Part model, mm, in its own coordinate system. A direction names the side the tool comes from. Give positions to 0.01 mm unless a question says otherwise; leave off trailing zeros. Order: outer loops, then holes, each group sorted by start corner. A loop starts at its lowest first (then second) coordinate and runs counter-clockwise, first axis right, second up. Notation, with made-up numbers: (39.25, 21) - (62.25, 21) arc R11 cw to (62.25, 27) - close; hole circle Ø9 at (85, -12.75). An arc over 180 degrees is marked (long way). One line per item, written item: value.
Autodesk Inventor part; units mm, degrees
ref_plane "YZ Plane" through (0, 0, 0) normal (1, 0, 0) x (0, 1, 0)
ref_plane "XZ Plane" through (0, 0, 0) normal (0, 1, 0) x (-1, 0, 0)
ref_plane "XY Plane" through (0, 0, 0) normal (0, 0, 1) x (1, 0, 0)
sketch "Sketch1" plane through (0, 0, 0) normal (0, 1, 0) x (-1, 0, 0)
  line L0 (18.2162, 77.2548) -> (-57.9838, 77.2548)
  line L1 (-57.9838, 77.2548) -> (-57.9838, -24.3452)
  line L2 (-57.9838, -24.3452) -> (18.2162, -24.3452)
  line L3 (18.2162, -24.3452) -> (18.2162, 77.2548)
  point P0 (0, 0)
  dimension "d0" = 101.6
  dimension "d1" = 76.2
extrude "Extrusion1" add sketch "Sketch1" along normal blind 12.7
sketch "Sketch2" plane through (57.9838, 0, -24.3452) normal (0, 0, -1) x (-1, 0, 0)
  line L0 (0, 0) -> (0, -203.2)
  line L1 (0, -203.2) -> (76.2, -203.2)
  line L2 (0, 0) -> (76.2, 0)
  line L3 (76.2, -203.2) -> (76.2, 0)
  line L4 (0, 12.7) -> (76.2, 12.7)
  line L5 (0, 0) -> (0, 12.7)
  line L6 (0, 12.7) -> (76.2, 12.7)
  line L7 (76.2, 12.7) -> (76.2, 0)
  point P0 (57.9838, 0)
  dimension "d4" = 90
  dimension "d5" = 203.2
extrude "Extrusion2" add sketch "Sketch2" along normal blind 12.7
sketch "Sketch3" plane through (-18.2162, 0, 77.2548) normal (0, 0, 1) x (1, 0, 0)
  line L0 (0, 0) -> (0, 12.7)
  line L1 (0, 0) -> (0, 12.7)
  line L2 (76.2, 0) -> (76.2, 12.7)
  line L3 (0, 12.7) -> (76.2, 12.7)
  line L4 (76.2, 12.7) -> (76.2, 0)
  line L5 (76.2, 0) -> (76.2, -203.2)
  line L6 (76.2, 0) -> (76.2, -203.2)
  line L7 (76.2, -203.2) -> (0, -203.2)
  line L8 (76.2, -203.2) -> (0, -203.2)
  line L9 (0, -203.2) -> (0, 0)
  point P0 (18.2162, 0)
extrude "Extrusion3" add sketch "Sketch3" along normal blind 12.7
sketch "Sketch4" plane through (0, 12.7, 0) normal (0, 1, 0) x (1, 0, 0)
  line L0 (-18.2162, -77.2548) -> (57.9838, -77.2548) construction
  line L1 (-18.2162, 24.3452) -> (-18.2162, -77.2548) construction
  line L2 (57.9838, -77.2548) -> (-18.2162, -77.2548) construction
  line L3 (-18.2162, -77.2548) -> (-18.2162, 24.3452) construction
  line L4 (-18.2162, 24.3452) -> (57.9838, 24.3452) construction
  line L5 (57.9838, 24.3452) -> (57.9838, -77.2548) construction
  line L6 (57.9838, 24.3452) -> (-18.2162, 24.3452) construction
  line L7 (-18.2162, -26.4548) -> (19.8838, -26.4548) construction
  line L8 (19.8838, -26.4548) -> (19.8838, 24.3452) construction
  line L9 (19.8838, 24.3452) -> (-18.2162, 24.3452) construction
  line L10 (-18.2162, 24.3452) -> (-18.2162, -26.4548) construction
  circle A0 centre (19.8838, -26.4548) radius 12.7
  dimension "d27" = 25.4
extrude "Extrusion4" add sketch "Sketch4" along normal blind 508
sketch "Sketch6" plane through (-18.2162, 0, 89.9548) normal (0, 0, 1) x (1, 0, 0)
  line L0 (0, -203.2) -> (76.2, -203.2) construction
  line L1 (38.1, -203.2) -> (76.2, -203.2) construction
  line L2 (76.2, -203.2) -> (76.2, -165.1) construction
  line L3 (76.2, -165.1) -> (38.1, -165.1) construction
  line L4 (38.1, -165.1) -> (38.1, -203.2) construction
  circle A0 centre (38.1, -165.1) radius 12.7
  point P0 (18.2162, 0)
  dimension "d28" = 25.4
extrude "Extrusion6" cut sketch "Sketch6" against normal through all
sketch "Sketch7" plane through (-18.2162, 0, 89.9548) normal (0, 0, 1) x (1, 0, 0)
  circle A0 centre (38.1, -165.1) radius 12.7 construction
  circle A1 centre (38.1, -165.1) radius 157.48 construction
  line L0 (38.1, -322.58) -> (38.1, -203.2) construction
  line L1 (0, -203.2) -> (76.2, -203.2) construction
  line L2 (0, 0) -> (0, -203.2) construction
  line L3 (0, -203.2) -> (38.1, -165.1) construction
  line L4 (76.2, -203.2) -> (76.2, 0) construction
  line L5 (38.1, -165.1) -> (76.2, -203.2) construction
  line L6 (38.1, -165.1) -> (0, -127) construction
  line L7 (38.1, -165.1) -> (76.2, -127) construction
  line L8 (12.7, -139.7) -> (63.5, -139.7) construction
  line L9 (63.5, -139.7) -> (63.5, -190.5) construction
  line L10 (63.5, -190.5) -> (12.7, -190.5) construction
  line L11 (12.7, -190.5) -> (12.7, -139.7) construction
  circle A2 centre (12.7, -139.7) radius 3.175
  circle A3 centre (63.5, -139.7) radius 3.175
  circle A4 centre (63.5, -190.5) radius 3.175
  circle A5 centre (12.7, -190.5) radius 3.175
  point P0 (18.2162, 0)
  dimension "d31" = 314.96
  dimension "d32" = 119.38
  dimension "d33" = 50.8
  dimension "d34" = 6.35
extrude "Extrusion7" cut sketch "Sketch7" against normal through all
properties part number "Big Wheel Mount"
1) Wall check: line 1 along X through (y, z) = (-190.5, 83.75); line 2 along X through (y, z) = (-139, -31); line 3 along Z through (x, y) = (19, -78). Give the ranges that are in metal, low to high. Write a range as [from, to].
Answer:
line 1: x = [-18.22, -8.69], [-2.34, 42.11], [48.46, 57.98]
line 2: x = [-18.22, -8.61], [-2.42, 42.19], [48.38, 57.98]
line 3: z = [-37.05, -24.35], [77.25, 89.95]
2) Slice it at B-B on y = -66. Write the cut outline in (x, z).
Answer:
outline: (-18.22, -37.05) - (57.98, -37.05) - (57.98, -24.35) - (-18.22, -24.35) - close; (-18.22, 77.25) - (57.98, 77.25) - (57.98, 89.95) - (-18.22, 89.95) - close
3) Drop flat-ended pins along their axis: P1, Ø8, axis at x = 28.5, z = 12.5, coming from the +Y side; P2, Ø5, axis at x = -9, z = 44.5, coming from the +Y side; P3, Ø8, axis at x = 21.5, z = 62.5, coming from the -Y side; P4, Ø4, axis at y = 432.5, z = 34, coming from the -X side. Give the stop position or say it passes through.
Answer:
P1: stops at y = 520.7
P2: stops at y = 12.7
P3: stops at y = 0
P4: stops at x = 8.46
4) Slice it at D-D on z = -8. Write the cut outline in (x, y).
Answer:
outline: (-18.22, 0) - (57.98, 0) - (57.98, 12.7) - (-18.22, 12.7) - close
5) Slice it at C-C on x = 16.5. Write the cut outline in (y, z).
Answer:
outline: (-203.2, -37.05) - (-177.34, -37.05) - (-177.34, -24.35) - (-203.2, -24.35) - close; (-203.2, 77.25) - (-177.34, 77.25) - (-177.34, 89.95) - (-203.2, 89.95) - close; (-152.86, -37.05) - (12.7, -37.05) - (12.7, 14.21) - (520.7, 14.21) - (520.7, 38.7) - (12.7, 38.7) - (12.7, 89.95) - (-152.86, 89.95) - (-152.86, 77.25) - (0, 77.25) - (0, -24.35) - (-152.86, -24.35) - close
6) Slice it at A-A on y = -165.1. Write the cut outline in (x, z), then the cut area to 3 significant figures.
Answer:
outline: (-18.22, -37.05) - (7.18, -37.05) - (7.18, -24.35) - (-18.22, -24.35) - close; (-18.22, 77.25) - (7.18, 77.25) - (7.18, 89.95) - (-18.22, 89.95) - close; (32.58, -37.05) - (57.98, -37.05) - (57.98, -24.35) - (32.58, -24.35) - close; (32.58, 77.25) - (57.98, 77.25) - (57.98, 89.95) - (32.58, 89.95) - close
area: 1,290 mm2
7) Two-plate mould, pull along Z, no slides. Class faces 4 (the face through (20, -203.2, -31)), 5 (the face through (19, -94, 89.955)), 6 (the face through (20, -100, -24.345)): pulls with the +Z half, pulls with the -Z half, needs draft (parallel to the pull), parting line crosses it, or undercut.
Answer:
face 4: needs draft
face 5: pulls with the +Z half
face 6: undercut
8) Which spindle directions (+Z, -Z, +X, -X, +Y, -Y) get a long thin tool onto all of the face, cutting with end or side? Do faces 1 (the face through (7.196, 263.144, 27.013)), 2 (the face through (-18.216, -72, 78)), 3 (the face through (20, 0, 27)). Say none if no direction does.
Answer:
face 1: +Y
face 2: +Z, -Z, -X, +Y, -Y
face 3: +X, -X, -Y
